Could you check a few things on this model? Use its own coordinates, in mm. Round coordinates to 2 decimals unless told otherwise and drop trailing zeros. Loops run counter-clockwise (first coordinate to the right, second up) from the corner with the lowest first, then second, coordinate; pieces in that order, holes last. Notation, with made-up numbers: (24, 43) -> (43, 43) arc R15 cw to (43, 51) -> close; hole circle Ø8 at (3, 47.5). An arc over 180 degrees is marked (long way). Put each result on its own line as item: value. Start each with the question number.
1. Imagine slicing it at D-D, the plane z = -35. Please give me the cut outline in (x, y).
2. Imagine slicing it at B-B, the plane y = 0.6. Please give me the cut outline in (x, z), and give its area (3 significant figures).
3. I'm going to push a flat-ended pin straight in: P1, Ø4, axis at x = 20, z = -30, coming from the -Y side. Where does the tip first touch, or does it pass through?
4. Imagine slicing it at A-A, the plane x = 50. Please give me the cut outline in (y, z).
5. If we mould it in two halves opening along Z, with no side actions, what happens to faces 1 (the cylindrical face through (6.014, 1.014, 34.297)), 2 (the cylindrical face through (74.297, 1.014, -33.986)), 3 (the cylindrical face through (22.48, 0.99, -10.33))? For each: pulls with the +Z half, pulls with the -Z half, needs draft (parallel to the pull), parting line crosses it, or undercut.
6. Imagine slicing it at C-C, the plane z = -11.5. Please give me the cut outline in (x, y).
7. I need wall thicknesses on line 1 (X direction, y = 0.65, z = -20); line 2 (X direction, y = 0.9, z = -0.5); line 3 (Z direction, x = 69, y = 0.9). Which ranges of each line are inside material? Lowest first, please. Write a range as [from, to].
```python
from build123d import *

# Parameters (mm, degrees)
SKETCH1_R           = 2.5
SKETCH1_W           = 40
SKETCH1_H           = 40
BOSS_EXTRUDE1_DEPTH = 2
FILLET1_R           = 50
FILLET2_R           = 20


with BuildPart() as part:
    # Sketch1 → Boss-Extrude1 (new body)
    # profile 1 of 2: a face of its own
    with BuildSketch(Plane(origin=(0, 0, 0), x_dir=(1, 0, 0), z_dir=(0, 1, 0))):
        Polygon((80, 0), (80, 40), (0, 40), (0, 0), (40, 0), align=None)
        with Locations(Location((20, 10, 0), (0, 0, 270))):
            Circle(SKETCH1_R, mode=Mode.SUBTRACT)
        with Locations(Location((20, 30, 0), (0, 0, 270))):
            Circle(SKETCH1_R, mode=Mode.SUBTRACT)
        with Locations(Location((50, 20, 0), (0, 0, 270))):
            Circle(SKETCH1_R, mode=Mode.SUBTRACT)
        with Locations(Location((65, 20, 0), (0, 0, 270))):
            Circle(SKETCH1_R, mode=Mode.SUBTRACT)
    # profile 2 of 2: a face of its own
    with BuildSketch(Plane(origin=(0, 0, 0), x_dir=(1, 0, 0), z_dir=(0, 1, 0))):
        with Locations((20, -20)):
            Rectangle(SKETCH1_W, SKETCH1_H)
        with Locations(Location((20, -20, 0), (0, 0, 270))):
            Circle(SKETCH1_R, mode=Mode.SUBTRACT)
    extrude(amount=BOSS_EXTRUDE1_DEPTH)

    # Fillet1
    # the kernel refuses this fillet: 50 mm, written as the material it adds along each edge
    with BuildSketch(Plane(origin=(40, 0, 0), x_dir=(0, 0, 1), z_dir=(0, 1, 0))) as fillet1_piece_1:
        with BuildLine():
            CenterArc((49.154759474, 49.154759474), FILLET1_R, 190.550098012, 68.899803976)
            Line((0, 40), (0, 0))
            Line((0, 0), (40, 0))
        make_face()
    extrude(amount=2)

    # Fillet2
    fillet2_edges = [part.edges().sort_by_distance(p)[0] for p in [
        (80, 1, -40),
        (80, 1, 0),
        (40, 1, 40),
        (0, 1, 40),
        (0, 1, -40),
    ]]
    fillet(fillet2_edges, radius=FILLET2_R)


solid = part.part
```
Entries:
1. outline: (6.77, 0) -> (73.23, 0) -> (73.23, 2) -> (6.77, 2) -> close
2. outline: (0, -20) arc R20 ccw to (20, -40) -> (60, -40) arc R20 ccw to (80, -20) -> (80, -14.48) arc R20 ccw to (68.33, 3.7) arc R50 cw to (43.7, 28.33) arc R20 ccw to (25.52, 40) -> (20, 40) arc R20 ccw to (0, 20) -> close; hole circle Ø5 at (20, -30); hole circle Ø5 at (20, -10); hole circle Ø5 at (20, 20); hole circle Ø5 at (50, -20); hole circle Ø5 at (65, -20)
2. area: 4,840 mm^2
3. P1: through
4. outline: (0, -40) -> (2, -40) -> (2, -22.5) -> (0, -22.5) -> close; (0, -17.5) -> (2, -17.5) -> (2, 18.06) -> (0, 18.06) -> close
5. face 1: pulls with the +Z half
5. face 2: pulls with the -Z half
5. face 3: undercut
6. outline: (0, 0) -> (18, 0) -> (18, 2) -> (0, 2) -> close; (22, 0) -> (79.78, 0) -> (79.78, 2) -> (22, 2) -> close
7. line 1: [0, 47.5], [52.5, 62.5], [67.5, 80]
7. line 2: [0, 74.3]
7. line 3: [-37.86, 3.38]
